Input: part model. Units: mm. Frame: model coordinates. A direction names the side the tool comes from. Give positions to 0.01 mm unless a question says otherwise; leave off trailing zeros. Order: outer loops, then holes, each group sorted by start corner. A loop starts at its lowest first (then second) coordinate and runs counter-clockwise, first axis right, second up. Notation, with made-up numbers: (70.25, -33) - (118.25, -33) arc R19 ccw to (118.25, 3) - close; hole circle Ø11 at (35, 85). An arc over 180 degrees is marked (long way). Answer in a Markdown table with one row per item. Add a question column.
from build123d import *

# Parameters (mm, degrees)
F1_DEPTH = 60
F3_DEPTH = 25
F4_R     = 5
F5_R     = 1.5


with BuildPart() as f1:
    # F0 (on Top) → F1 (new body)
    with BuildSketch(Plane.XY):
        Polygon((-20.3012, 115.696498), (-27.3, 115.56689), (-27.3, -64.43311), (-20.3, -64.43311), (-20.3, -29.43311), (-7, -29.43311), (-7, -64.43311), (0, -64.43311), (0, -22.43311), (-20.3012, -22.43311), align=None)
    extrude(amount=F1_DEPTH)

    # F2 (on face) → F3 (cut)
    with BuildSketch(Plane.YZ.offset(-20.3012)):
        Polygon((32.132399, 30), (-12.43311, 45.757328), (-12.43311, 14.242672), align=None)
        Polygon((88.697203, 50), (-0.433815, 50), (44.131694, 34.242672), align=None)
        Polygon((100.696498, 14.242672), (100.696498, 45.757328), (56.130989, 30), align=None)
        Polygon((44.131694, 25.757328), (-0.433815, 10), (88.697203, 10), align=None)
    extrude(amount=-F3_DEPTH, mode=Mode.SUBTRACT)

    # F4
    f4_edges = [f1.edges().sort_by_distance(p)[0] for p in [
        (0, -22.43311, 30),
        (-20.3012, -22.43311, 30),
    ]]
    fillet(f4_edges, radius=F4_R)

    # F5
    f5_edges = [f1.edges().sort_by_distance(p)[0] for p in [
        (-23.8006, -12.43311, 14.242672),
        (-23.8006, -12.43311, 45.757328),
        (-23.8006, -0.433815, 10),
        (-23.8006, -0.433815, 50),
        (-23.8006, 32.132399, 30),
        (-23.8006, 44.131694, 34.242672),
        (-23.8006, 44.131694, 25.757328),
        (-23.8006, 56.130989, 30),
        (-23.8006, 88.697203, 50),
        (-23.8006, 100.696498, 45.757328),
        (-23.8006, 100.696498, 14.242672),
        (-23.8006, 88.697203, 10),
    ]]
    fillet(f5_edges, radius=F5_R)


solid = f1.part
Q1. Section B-B, the plane z = 54. Return loops of the section in (x, y).
Q2. Contact query for flat-ended pins moving along their axis: P1, Ø5, axis at x = -4, z = 12.5, coming from the +Y side; P2, Ø2, axis at x = -18, z = 19.5, coming from the -Y side; P3, Ø1.5, axis at x = -23.5, z = 44.5, coming from the +Y side. Output: stop coordinate, or through.
Q3. Line query: probe 1 along X at (y, z) = (-49, 35.5); probe 2 along Y at (x, z) = (-21, 2); probe 3 along Z at (x, y) = (-20.5, 58.5). Output: solid intervals per line, ascending.
Q4. Section C-C, the plane y = 55.5. Return loops of the section in (x, z), then the cut area to 3 significant figures.
Q5. Pull-direction query (X, two-part tool) for faces 4 (the flat face through (-7, -47, 30)), 5 (the flat face through (-21, 6, 0)), 6 (the flat face through (-20.301, 48, 30)); classes: +X half, -X half, draft (parallel to the pull), parting line (faces both ways), or undercut.
Q6. Section A-A, the plane y = -52. Return loops of the section in (x, z).
Q7. Access query for faces 1 (the flat face through (-21, 6, 60)), 2 (the flat face through (-24, -12.433, 30)), 3 (the flat face through (-10, -22.433, 30)). Directions: +Z, -Z, +X, -X, +Y, -Y. A direction counts if a zero-diameter tool reaches every point of the face in a straight line with its end or side. Return the directions, or none.
Q8. Section D-D, the plane x = -22. Return loops of the section in (y, z).
Computed:
| question | item | result |
|---|---|---|
| 1 | outline | (-27.3, -64.43) - (-20.3, -64.43) - (-20.3, -29.43) - (-7, -29.43) - (-7, -64.43) - (0, -64.43) - (0, -27.43) arc R5 ccw to (-5, -22.43) - (-15.3, -22.43) arc R5 cw to (-20.3, -17.43) - (-20.3, 115.7) - (-27.3, 115.57) - close |
| 2 | P1 | stops at y = -22.43 |
| 2 | P2 | stops at y = -29.43 |
| 2 | P3 | stops at y = 115.65 |
| 3 | probe 1 | x = -27.3 to -20.3, -7 to 0 |
| 3 | probe 2 | y = -64.43 to 115.68 |
| 3 | probe 3 | z = 0 to 10, 20.68 to 39.32, 50 to 60 |
| 4 | outline | (-27.3, 0) - (-20.3, 0) - (-20.3, 10) - (-27.3, 10) - close; (-27.3, 21.74) - (-20.3, 21.74) - (-20.3, 38.26) - (-27.3, 38.26) - close; (-27.3, 50) - (-20.3, 50) - (-20.3, 60) - (-27.3, 60) - close |
| 4 | area | 256 mm^2 |
| 5 | face 4 | undercut |
| 5 | face 5 | draft |
| 5 | face 6 | +X half |
| 6 | outline | (-27.3, 0) - (-20.3, 0) - (-20.3, 60) - (-27.3, 60) - close; (-7, 0) - (0, 0) - (0, 60) - (-7, 60) - close |
| 7 | face 1 | +Z, +X, -X, +Y, -Y |
| 7 | face 2 | +X, -X |
| 7 | face 3 | +Z, -Z, +X, +Y |
| 8 | outline | (-64.43, 0) - (115.67, 0) - (115.67, 60) - (-64.43, 60) - close; hole (-12.43, 16.36) arc R1.5 ccw to (-10.43, 14.95) - (28.13, 28.59) arc R1.5 ccw to (28.13, 31.41) - (-10.43, 45.05) arc R1.5 ccw to (-12.43, 43.64) - close; hole (7.81, 12.91) arc R1.5 ccw to (8.31, 10) - (79.96, 10) arc R1.5 ccw to (80.46, 12.91) - (44.63, 25.58) arc R1.5 ccw to (43.63, 25.58) - close; hole (7.81, 47.09) - (43.63, 34.42) arc R1.5 ccw to (44.63, 34.42) - (80.46, 47.09) arc R1.5 ccw to (79.96, 50) - (8.31, 50) arc R1.5 ccw to start; hole (60.13, 28.59) - (98.7, 14.95) arc R1.5 ccw to (100.7, 16.36) - (100.7, 43.64) arc R1.5 ccw to (98.7, 45.05) - (60.13, 31.41) arc R1.5 ccw to start |
